```python
from build123d import *

# Parameters (mm, degrees)
SKETCH022_R     = 1.6
PAD008_DEPTH    = 4
PAD009_DEPTH    = 18
SKETCH024_R     = 2.5
POCKET014_DEPTH = 6.5
SKETCH025_R     = 1.6
POCKET015_DEPTH = 5
POCKET020_DEPTH = 5
SKETCH038_W     = 11
SKETCH038_H     = 4.9
POCKET024_DEPTH = 3.5


with BuildPart() as part:
    # Sketch022 (on ShapeBinder) → Pad008 (new body)
    with BuildSketch(Plane(origin=(0, 0, -95), x_dir=(1, 0, 0), z_dir=(0, 0, -1))):
        with BuildLine():
            Line((-126, 55), (126, 55))
            ThreePointArc((130, 51), (128.828427, 53.828427), (126, 55))
            Line((130, -51), (130, 51))
            ThreePointArc((126, -55), (128.828427, -53.828427), (130, -51))
            Line((-126, -55), (126, -55))
            ThreePointArc((-130, -51), (-128.828427, -53.828427), (-126, -55))
            Line((-130, 51), (-130, -51))
            ThreePointArc((-126, 55), (-128.828427, 53.828427), (-130, 51))
        make_face()
        with Locations((124, 49)):
            Circle(SKETCH022_R, mode=Mode.SUBTRACT)
        with Locations((124, -49)):
            Circle(SKETCH022_R, mode=Mode.SUBTRACT)
        with Locations((44, -48.010154)):
            Circle(SKETCH022_R, mode=Mode.SUBTRACT)
        with Locations((-44, -48.010154)):
            Circle(SKETCH022_R, mode=Mode.SUBTRACT)
        with Locations((-124, -49)):
            Circle(SKETCH022_R, mode=Mode.SUBTRACT)
        with Locations((-124, 49)):
            Circle(SKETCH022_R, mode=Mode.SUBTRACT)
        with Locations((-55.592233, 48.010154)):
            Circle(SKETCH022_R, mode=Mode.SUBTRACT)
        with Locations((55.592233, 48.010154)):
            Circle(SKETCH022_R, mode=Mode.SUBTRACT)
        with BuildLine():
            ThreePointArc((-95, -33), (-97, -35), (-95, -37))
            Line((-95, -37), (-85, -37))
            ThreePointArc((-85, -37), (-83, -35), (-85, -33))
            Line((-95, -33), (-85, -33))
        make_face(mode=Mode.SUBTRACT)
        with BuildLine():
            ThreePointArc((-5, -33), (-7, -35), (-5, -37))
            Line((-5, -37), (5, -37))
            ThreePointArc((5, -37), (7, -35), (5, -33))
            Line((-5, -33), (5, -33))
        make_face(mode=Mode.SUBTRACT)
        with BuildLine():
            ThreePointArc((85, -33), (83, -35), (85, -37))
            Line((85, -37), (95, -37))
            ThreePointArc((95, -37), (97, -35), (95, -33))
            Line((85, -33), (95, -33))
        make_face(mode=Mode.SUBTRACT)
    extrude(amount=PAD008_DEPTH)

    # Sketch023 (on Face30 of Pad008) → Pad009 (join)
    with BuildSketch(Plane(origin=(0, 0, -99), x_dir=(1, 0, 0), z_dir=(0, 0, -1))):
        with BuildLine():
            Line((-126, 55), (126, 55))
            ThreePointArc((130, 51), (128.828427, 53.828427), (126, 55))
            Line((130, 51), (130, -51))
            ThreePointArc((126, -55), (128.828427, -53.828427), (130, -51))
            Line((126, -55), (-126, -55))
            ThreePointArc((-130, -51), (-128.828427, -53.828427), (-126, -55))
            Line((-130, -51), (-130, 51))
            ThreePointArc((-126, 55), (-128.828427, 53.828427), (-130, 51))
        make_face()
        with BuildLine():
            ThreePointArc((-46.245109, -50), (-44, -51.010154), (-41.754891, -50))
            Line((-41.754891, -50), (-5, -50))
            ThreePointArc((5, -50), (0, -45), (-5, -50))
            Line((41.754891, -50), (5, -50))
            ThreePointArc((41.754891, -50), (44, -51.010154), (46.245109, -50))
            Line((46.245109, -50), (106.171573, -50))
            ThreePointArc((116.171573, -50), (111.171573, -45), (106.171573, -50))
            Line((121.171573, -50), (116.171573, -50))
            ThreePointArc((121.171573, -50), (126.12132, -51.12132), (125, -46.171573))
            Line((125, -46.171573), (125, -5))
            ThreePointArc((125, 5), (120, 0), (125, -5))
            Line((125, 46.171573), (125, 5))
            ThreePointArc((125, 46.171573), (126.12132, 51.12132), (121.171573, 50))
            Line((121.171573, 50), (116.171573, 50))
            ThreePointArc((106.171573, 50), (111.171573, 45), (116.171573, 50))
            Line((57.837342, 50), (106.171573, 50))
            ThreePointArc((57.837342, 50), (55.592233, 51.010154), (53.347124, 50))
            Line((53.347124, 50), (5, 50))
            ThreePointArc((-5, 50), (0, 45), (5, 50))
            Line((-53.347124, 50), (-5, 50))
            ThreePointArc((-53.347124, 50), (-55.592233, 51.010154), (-57.837342, 50))
            Line((-57.837342, 50), (-106.171573, 50))
            ThreePointArc((-116.171573, 50), (-111.171573, 45), (-106.171573, 50))
            Line((-121.171573, 50), (-116.171573, 50))
            ThreePointArc((-121.171573, 50), (-126.12132, 51.12132), (-125, 46.171573))
            Line((-125, 46.171573), (-125, 5))
            ThreePointArc((-125, -5), (-120, 0), (-125, 5))
            Line((-125, -46.171573), (-125, -5))
            ThreePointArc((-125, -46.171573), (-126.12132, -51.12132), (-121.171573, -50))
            Line((-121.171573, -50), (-116.171573, -50))
            ThreePointArc((-106.171573, -50), (-111.171573, -45), (-116.171573, -50))
            Line((-46.245109, -50), (-106.171573, -50))
        make_face(mode=Mode.SUBTRACT)
    extrude(amount=PAD009_DEPTH)

    # Sketch024 (on Face33 of Pad009) → Pocket014 (cut)
    with BuildSketch(Plane(origin=(0, 0, -117), x_dir=(1, 0, 0), z_dir=(0, 0, -1))):
        with Locations((-111.171573, 50)):
            Circle(SKETCH024_R)
        with Locations((0, 50)):
            Circle(SKETCH024_R)
        with Locations((111.171573, 50)):
            Circle(SKETCH024_R)
        with Locations((-125, 0)):
            Circle(SKETCH024_R)
        with Locations((-111.171573, -50)):
            Circle(SKETCH024_R)
        with Locations((0, -50)):
            Circle(SKETCH024_R)
        with Locations((111.171573, -50)):
            Circle(SKETCH024_R)
        with Locations((125, 0)):
            Circle(SKETCH024_R)
    extrude(amount=-POCKET014_DEPTH, mode=Mode.SUBTRACT)

    # Sketch025 (on Face83 of Pocket014) → Pocket015 (cut)
    with BuildSketch(Plane(origin=(0, 0, -110.5), x_dir=(1, 0, 0), z_dir=(0, 0, -1))):
        with Locations((0, -50)):
            Circle(SKETCH025_R)
        with Locations((-125, 0)):
            Circle(SKETCH025_R)
        with Locations((111.171573, -50)):
            Circle(SKETCH025_R)
        with Locations((-111.171573, -50)):
            Circle(SKETCH025_R)
        with Locations((57.837342, 50)):
            Circle(SKETCH025_R)
        with Locations((125, 0)):
            Circle(SKETCH025_R)
        with Locations((0, 50)):
            Circle(SKETCH025_R)
        with Locations((111.171573, 50)):
            Circle(SKETCH025_R)
    extrude(amount=-POCKET015_DEPTH, mode=Mode.SUBTRACT)

    # Sketch032 (on Face9 of Pocket015) → Pocket020 (cut)
    with BuildSketch(Plane(origin=(-130, 0, 0), x_dir=(0, -1, 0), z_dir=(-1, 0, 0))):
        with BuildLine():
            ThreePointArc((34.3, -103.9), (36, -102.2), (34.3, -100.5))
            Line((34.3, -100.5), (28.6, -100.5))
            ThreePointArc((28.6, -100.5), (26.9, -102.2), (28.6, -103.9))
            Line((34.3, -103.9), (28.6, -103.9))
        make_face()
    extrude(amount=-POCKET020_DEPTH, mode=Mode.SUBTRACT)

    # Sketch038 (on Face62 of Pocket020) → Pocket024 (cut)
    with BuildSketch(Plane.YZ.offset(-125)):
        with Locations((-31.45, -101.45)):
            Rectangle(SKETCH038_W, SKETCH038_H)
    extrude(amount=-POCKET024_DEPTH, mode=Mode.SUBTRACT)


solid = part.part
```
For this review, take the finished solid that the model builds, in its own axes (mm). Coordinates: 2 decimals unless noted, no trailing zeros. Order: outer loops, then holes, each group sorted by start corner. A loop starts at its lowest first (then second) coordinate and runs counter-clockwise, first axis right, second up. Notation, with made-up numbers: (81.5, 36.5) -> (108.5, 36.5) arc R4 ccw to (108.5, 42.5) -> close; hole circle Ø1 at (-0.75, 70). An arc over 180 degrees is marked (long way). Use CSV: the item, a comma, the result in double quotes. Start each with the question number.
Item 1: We need section C-C, the plane z = -114. Give the number of separate pieces and of enclosed holes in the cut face, then the cut area to 3 significant figures.
Item 2: Wall thickness on probe 1 along X at (y, z) = (0, -109.2); probe 2 along Y at (x, z) = (0, -108.55); probe 3 along Y at (x, z) = (-124, -106.5): over which ranges is each line inside the solid? List them lowest first.
Item 3: We need section A-A, the plane x = 90.5. Give the boundary of the cut face in (y, z), then the cut area to 3 significant figures.
Item 4: Insertion check: pin 1 (12 mm diameter, centred on x = -7, y = 39, fed in from -Z); pin 2 (3.5 mm diameter, centred on x = 0, y = 50.5, fed in from -Z); pin 3 (3 mm diameter, centred on x = -111.17, y = 50, fed in from -Z). Each pin has a flat end and moves straight along its axis. Give the tip position at first contact, or say it passes through.
Item 5: We need section D-D, the plane x = 49. Give the boundary of the cut face in (y, z).
Item 6: We need section B-B, the plane y = 11. Give the boundary of the cut face in (x, z).
Derived:
1,separate pieces,"1"
1,enclosed holes,"9"
1,area,"3,670 mm^2"
2,probe 1,"x = -130 to -126.6, -123.4 to -120, 120 to 123.4, 126.6 to 130"
2,probe 2,"y = -55 to -51.6, -48.4 to -45, 45 to 48.4, 51.6 to 55"
2,probe 3,"y = -55 to -52, -4.9 to -1.25, 1.25 to 4.9, 52 to 55"
3,outline,"(-55, -117) -> (-50, -117) -> (-50, -99) -> (33, -99) -> (33, -95) -> (-55, -95) -> close; (37, -99) -> (50, -99) -> (50, -117) -> (55, -117) -> (55, -95) -> (37, -95) -> close"
3,area,"604 mm^2"
4,pin 1,"stops at z = -99"
4,pin 2,"stops at z = -110.5"
4,pin 3,"stops at z = -105.5"
5,outline,"(-55, -117) -> (-50, -117) -> (-50, -99) -> (50, -99) -> (50, -117) -> (55, -117) -> (55, -95) -> (-55, -95) -> close"
6,outline,"(-130, -117) -> (-125, -117) -> (-125, -99) -> (125, -99) -> (125, -117) -> (130, -117) -> (130, -95) -> (-130, -95) -> close"
